```python
from build123d import *

# Parameters (mm, degrees)
SKETCH_2_W           = 150
SKETCH_2_H           = 43
SKETCH_2_R           = 4.05
EXTRUDE_1_DEPTH      = 8
SKETCH_3_R           = 2.55
CUT_EXTRUDE_1_DEPTH  = 157.246599963
CUT_EXTRUDE_16_DEPTH = 6
CUT_EXTRUDE_2_DEPTH  = 157.246599963
SKETCH_25_R          = 1.55
CUT_EXTRUDE_13_DEPTH = 157.246599963
CUT_EXTRUDE_11_DEPTH = 2
EXTRUDE_2_DEPTH      = 8


with BuildPart() as part:
    # 草图2 → 凸台-拉伸1 (new body)
    with BuildSketch(Plane.XY):
        with Locations((75, 21.5)):
            Rectangle(SKETCH_2_W, SKETCH_2_H)
        with Locations((7, 8)):
            Circle(SKETCH_2_R, mode=Mode.SUBTRACT)
        with Locations((75, 10)):
            Circle(SKETCH_2_R, mode=Mode.SUBTRACT)
        with Locations((143, 8)):
            Circle(SKETCH_2_R, mode=Mode.SUBTRACT)
    extrude_1 = extrude(amount=EXTRUDE_1_DEPTH)

    # 草图3 → 切除-拉伸1 (cut, through all)
    with BuildSketch(Plane.XY.offset(8)):
        with Locations((23, 8)):
            Circle(SKETCH_3_R)
        with Locations((127, 8)):
            Circle(SKETCH_3_R)
    cut_extrude_1 = extrude(amount=-CUT_EXTRUDE_1_DEPTH, mode=Mode.SUBTRACT)

    # 草图28 → 切除-拉伸16 (cut)
    with BuildSketch(Plane(origin=(0, 0, 0), x_dir=(-1, 0, 0), z_dir=(0, 0, -1))):
        Polygon((-122.9, 5.632863896), (-122.9, 10.367136104), (-127, 12.734272207), (-131.1, 10.367136104), (-131.1, 5.632863896), (-127, 3.265727793), align=None)
        Polygon((-18.9, 5.632863896), (-18.9, 10.367136104), (-23, 12.734272207), (-27.1, 10.367136104), (-27.1, 5.632863896), (-23, 3.265727793), align=None)
    cut_extrude_16 = extrude(amount=-CUT_EXTRUDE_16_DEPTH, mode=Mode.SUBTRACT)

    # 草图4 → 切除-拉伸2 (cut, through all)
    with BuildSketch(Plane(origin=(150, 0, 0), x_dir=(0, 0, -1), z_dir=(1, 0, 0))):
        Polygon((-1.5, 41.2), (-2.5, 41.2), (-2.5, 43), (0, 43), (0, 37.8), (-1.5, 37.8), align=None)
    cut_extrude_2 = extrude(amount=-CUT_EXTRUDE_2_DEPTH, mode=Mode.SUBTRACT)

    # 草图25 → 切除-拉伸13 (cut, through all)
    with BuildSketch(Plane(origin=(0, 0, 0), x_dir=(-1, 0, 0), z_dir=(0, 0, -1))):
        with Locations((-130, 34)):
            Circle(SKETCH_25_R)
        with Locations((-20, 34)):
            Circle(SKETCH_25_R)
    cut_extrude_13 = extrude(amount=-CUT_EXTRUDE_13_DEPTH, mode=Mode.SUBTRACT)

    # 草图19 → 切除-拉伸11 (cut)
    with BuildSketch(Plane(origin=(0, 0, 2.5), x_dir=(-1, 0, 0), z_dir=(0, 0, -1))):
        with BuildLine():
            Line((-60, 43), (-90.247938178, 43))
            Line((-90.247938178, 43), (-90.247938178, 42.2))
            ThreePointArc((-90.247938178, 42.2), (-89.747938178, 41.7), (-89.247938178, 42.2))
            Line((-89.247938178, 42.2), (-61, 42.2))
            ThreePointArc((-61, 42.2), (-60.5, 41.7), (-60, 42.2))
            Line((-60, 42.2), (-60, 43))
        make_face()
    cut_extrude_11 = extrude(amount=-CUT_EXTRUDE_11_DEPTH, mode=Mode.SUBTRACT)

    # 草图22 → 凸台-拉伸2 (add)
    with BuildSketch(Plane.XY.offset(8)):
        with BuildLine():
            Line((0, -4), (5.5, -4))
            ThreePointArc((5.5, -4), (3.5, -2), (5.5, 0))
            Line((5.5, 0), (0, 0))
            ThreePointArc((0, 0), (2, -2), (0, -4))
        make_face()
        with BuildLine():
            Line((150, 0), (144.5, 0))
            ThreePointArc((144.5, 0), (146.5, -2), (144.5, -4))
            Line((144.5, -4), (150, -4))
            ThreePointArc((150, -4), (148, -2), (150, 0))
        make_face()
    extrude(amount=-EXTRUDE_2_DEPTH)

    # 镜向2: 凸台-拉伸1, 切除-拉伸1, 切除-拉伸16, 切除-拉伸2, 切除-拉伸13, 切除-拉伸11 across plane
    add(extrude_1.mirror(Plane(origin=(0, -1.9, 0), x_dir=(0, 0, 1), z_dir=(0, -1, 0))))
    add(cut_extrude_1.mirror(Plane(origin=(0, -1.9, 0), x_dir=(0, 0, 1), z_dir=(0, -1, 0))), mode=Mode.SUBTRACT)
    add(cut_extrude_16.mirror(Plane(origin=(0, -1.9, 0), x_dir=(0, 0, 1), z_dir=(0, -1, 0))), mode=Mode.SUBTRACT)
    add(cut_extrude_2.mirror(Plane(origin=(0, -1.9, 0), x_dir=(0, 0, 1), z_dir=(0, -1, 0))), mode=Mode.SUBTRACT)
    add(cut_extrude_13.mirror(Plane(origin=(0, -1.9, 0), x_dir=(0, 0, 1), z_dir=(0, -1, 0))), mode=Mode.SUBTRACT)
    add(cut_extrude_11.mirror(Plane(origin=(0, -1.9, 0), x_dir=(0, 0, 1), z_dir=(0, -1, 0))), mode=Mode.SUBTRACT)


solid = part.part
```
Build history of the part. All positions in model axes, mm. A direction names the side the tool comes from. Give positions to 0.01 mm unless a question says otherwise; leave off trailing zeros. Order: outer loops, then holes, each group sorted by start corner. A loop starts at its lowest first (then second) coordinate and runs counter-clockwise, first axis right, second up. Notation, with made-up numbers: M 31,-23 L 49,-23 A22 ccw 49,-3 Z; hole C -24,87.25 d2. An arc over 180 degrees is marked long. Return JSON: item names as keys, results as strings.
Q1. 3-axis set-ups, long thin cutter, end or side, ignore diameter. For faces 1 (the face through (74, 0, 4)), 2 (the face through (0, 21, 4)), 3 (the face through (122.9, -12, 3)): which of +Z, -Z, +X, -X, +Y, -Y reach the whole face in a straight line?
Answer list:
{"face 1": "+Z, -Z", "face 2": "+Z, -Z, -X, +Y, -Y", "face 3": "-Z"}
Q2. Band-saw the part on A-A (x = 31). Give the cut face in (y, z), then the cut area to 3 significant figures.
Answer list:
{"outline": "M -46.8,2.5 L -45,2.5 L -45,1.5 L -41.6,1.5 L -41.6,0 L -3.8,0 L -3.8,8 L -46.8,8 Z; M 0,0 L 37.8,0 L 37.8,1.5 L 41.2,1.5 L 41.2,2.5 L 43,2.5 L 43,8 L 0,8 Z", "area": "669 mm^2"}
Q3. Wall check: probe 1 along Y at (x, z) = (143, 5); probe 2 along Y at (x, z) = (127, 6.6); probe 3 along Y at (x, z) = (108.5, 6.5). Give the ranges that are in metal, low to high. Write a range as from..to.
Answer list:
{"probe 1": "y = -46.8..-15.85, -7.75..-3.8, 0..3.95, 12.05..43", "probe 2": "y = -46.8..-14.35, -9.25..-3.8, 0..5.45, 10.55..43", "probe 3": "y = -46.8..-3.8, 0..43"}
Q4. Band-saw the part on B-B (y = -37.8). Give the cut face in (x, z).
Answer list:
{"outline": "M 0,0 L 18.45,0 L 18.45,8 L 0,8 Z; M 21.55,0 L 128.45,0 L 128.45,8 L 21.55,8 Z; M 131.55,0 L 150,0 L 150,8 L 131.55,8 Z"}
Q5. Band-saw the part on C-C (x = 143). Give the cut face in (y, z), then the cut area to 3 significant figures.
Answer list:
{"outline": "M -46.8,2.5 L -45,2.5 L -45,1.5 L -41.6,1.5 L -41.6,0 L -15.85,0 L -15.85,8 L -46.8,8 Z; M -7.75,0 L -3.8,0 L -3.8,8 L -7.75,8 Z; M 0,0 L 3.95,0 L 3.95,8 L 0,8 Z; M 12.05,0 L 37.8,0 L 37.8,1.5 L 41.2,1.5 L 41.2,2.5 L 43,2.5 L 43,8 L 12.05,8 Z", "area": "539 mm^2"}
Q6. Band-saw the part on D-D (y = -11.8). Count the separate pieces of the cut face and the enclosed holes in it, then the cut area to 3 significant figures.
Answer list:
{"separate pieces": "6", "enclosed holes": "0", "area": "895 mm^2"}
Q7. Two-plate mould, pull along Y, no slides. Class faces 4 (the face through (76, -43, 1.5)), 5 (the face through (25.079, 4.466, 2.958)): pulls with the +Y half, pulls with the -Y half, needs draft (parallel to the pull), parting line crosses it, or undercut.
Answer list:
{"face 4": "needs draft", "face 5": "undercut"}
Q8. Flat gauge pins, fed straight in: pin 1 (3 mm diameter, centred on x = 70.5, z = 2, fed in from +Y); pin 2 (1.4 mm diameter, centred on x = 67.5, y = 42, fed in from -Z); pin 3 (0.5 mm diameter, centred on x = 102.5, z = 2, fed in from -Y). Where does each tip first touch, or does it go through?
Answer list:
{"pin 1": "stops at y = 42.2", "pin 2": "stops at z = 2.5", "pin 3": "stops at y = -45"}
